Input: part model. Units: mm. Frame: model coordinates. Face numbers are marked on the shaded views. Give positions to 0.01 mm unless a question says otherwise; leave off trailing zeros. Loops run counter-clockwise (first coordinate to the right, second up) from the corner with the lowest first, then second, coordinate; pieces in that order, holes last. Notation, with made-up numbers: M 52,77.25 L 70,77.25 A17 ccw 70,101.25 Z; hole C -37.5,77 d10. An arc over 180 degrees is marked long. Use CSV: the item, a comma, the result in double quotes. Start each with the question number.
from build123d import *

# Parameters (mm, degrees)
F0_W     = 38.7298334621
F0_H     = 10
F1_DEPTH = 10
F3_DEPTH = 41
F4_F1_R  = 0.5
F4_F2_R  = 0.5


with BuildPart() as f1:
    # F0 (on Top) → F1 (new body)
    with BuildSketch(Plane.XY):
        with BuildLine():
            Line((-19.364916731, 5), (19.364916731, 5))
            ThreePointArc((19.364916731, 5), (0, 20), (-19.364916731, 5))
        make_face()
        Rectangle(F0_W, F0_H)
        with BuildLine():
            ThreePointArc((-19.364916731, -5), (0, -20), (19.364916731, -5))
            Line((19.364916731, -5), (-19.364916731, -5))
        make_face()
        with BuildLine():
            Line((-19.364916731, -5), (-19.364916731, 5))
            ThreePointArc((-19.364916731, 5), (-20, 0), (-19.364916731, -5))
        make_face()
    extrude(amount=-F1_DEPTH)

    # F2 (on face) → F3 (join)
    with BuildSketch(Plane.XY):
        with BuildLine():
            ThreePointArc((-12.8038080273, 2.25), (0, 13), (12.8038080273, 2.25))
            Line((12.8038080273, 2.25), (14.3243673508, 2.25))
            ThreePointArc((14.3243673508, 2.25), (0, 14.5), (-14.3243673508, 2.25))
            Line((-14.3243673508, 2.25), (-12.8038080273, 2.25))
        make_face()
        with BuildLine():
            Line((14.3243673508, -2.25), (12.8038080273, -2.25))
            ThreePointArc((12.8038080273, -2.25), (0, -13), (-12.8038080273, -2.25))
            Line((-12.8038080273, -2.25), (-14.3243673508, -2.25))
            ThreePointArc((-14.3243673508, -2.25), (0, -14.5), (14.3243673508, -2.25))
        make_face()
        with BuildLine():
            ThreePointArc((-12.8038080273, -2.25), (-13, 0), (-12.8038080273, 2.25))
            Line((-12.8038080273, 2.25), (-14.3243673508, 2.25))
            ThreePointArc((-14.3243673508, 2.25), (-14.5, 0), (-14.3243673508, -2.25))
            Line((-14.3243673508, -2.25), (-12.8038080273, -2.25))
        make_face()
    extrude(amount=F3_DEPTH)

    # F4: fillet of radius 0.5 on 7 edges, made by hand

    # F4_f1
    f4_f1_edges = [f1.edges().sort_by_distance(p)[0] for p in [
        (-20, 0, 0),
        (12.8038080273, 2.25, 20.5),
        (12.8038080273, -2.25, 20.5),
        (14.3243673508, 2.25, 20.5),
        (14.3243673508, -2.25, 20.5),
    ]]
    fillet(f4_f1_edges, radius=F4_F1_R)

    # F4_f2
    f4_f2_edges = [f1.edges().sort_by_distance(p)[0] for p in [
        (-14.5, 0, 0),
        (-13, 0, 0),
        (12.9014449798, -2.3621044432, 0),
        (12.9014449798, 2.3621044432, 0),
        (14.1139754816, 2.4330671545, 0),
        (14.1139754816, -2.4330671545, 0),
    ]]
    fillet(f4_f2_edges, radius=F4_F2_R)


solid = f1.part
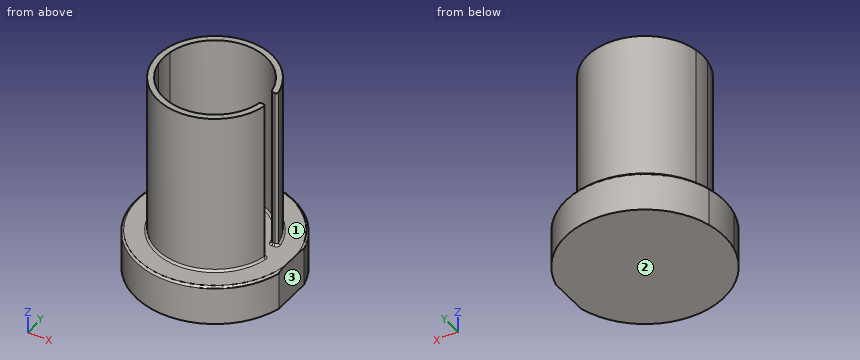
Item 1: Mould query, pull axis X, two halves, no side actions, for the marked faces 1, 2 and 3. Classes: +X half, -X half, draft (parallel to the pull), parting line (faces both ways), or undercut.
Item 2: First-contact query: pin 1 Ø8 at (y, z) = (-11, -4.5) entering from +X (3 decimals); pin 2 Ø11.5 at (x, y) = (-0.5, 3.5) entering from +Z; pin 3 Ø0.6 at (x, z) = (13.5, 24.5) entering from +Y; pin 4 Ø6 at (x, z) = (1.5, 1.5) entering from -Y. Flat tips, straight axial feed; report the tip coordinate or a pass-through.
Item 3: Section B-B (z = -5). Output: boundary loops of the cut face in (x, y), then the cut area to 3 significant figures.
Item 4: Material intervals for line 1 (X direction, y = 12, z = 25.5); line 2 (Z direction, x = 2.5, y = -5.5); line 3 (X direction, y = -7, z = 36.5), sorted ascending.
Item 5: Section A-A (z = 26). Output: boundary loops of the cut face in (x, y), then the cut area to 3 significant figures.
Recorded:
1,face 1,"undercut"
1,face 2,"draft"
1,face 3,"+X half"
2,pin 1,"x = 18.735"
2,pin 2,"z = 0"
2,pin 3,"y = 6"
2,pin 4,"y = -20"
3,outline,"M 19.36,-5 L 19.36,5 A20 ccw long Z"
3,area,"1,250 mm²"
4,line 1,"-8.14 to -5, 5 to 8.14"
4,line 2,"-10 to 0"
4,line 3,"-12.7 to -10.95, 10.95 to 12.7"
5,outline,"M 12.73,-2.65 A13 cw long 12.73,2.65 A0.5 ccw 13.22,2.25 L 13.73,2.25 A0.5 ccw 14.22,2.85 A14.5 ccw long 14.22,-2.85 A0.5 ccw 13.73,-2.25 L 13.22,-2.25 A0.5 ccw Z"
5,area,"123 mm²"
